Read the model definition and answer for the solid it produces. Units are mm, in the model's axes. Give positions to 0.01 mm unless a question says otherwise; leave off trailing zeros. Order: outer loops, then holes, each group sorted by start corner. A loop starts at its lowest first (then second) coordinate and runs counter-clockwise, first axis right, second up.
Item 1: A cutting plane is placed at D-D (z = 13.3). Write down the section's boundary in (x, y), plus the area to 3 significant figures.
Item 2: A cutting plane is placed at C-C (y = 2). Write down the section's boundary in (x, z), plus the area to 3 significant figures.
Item 3: The mould has two halves that part along Y. Classify faces 1 (the face through (0, -6, 10)), 2 (the face through (13.32, -9.74, 11.01)): +Y half, -Y half, draft (parallel to the pull), parting line (faces both ways), or undercut.
Item 4: A cutting plane is placed at B-B (x = -13.5). Write down the section's boundary in (y, z).
Item 5: A cutting plane is placed at A-A (x = 0). Write down the section's boundary in (y, z), plus the area to 3 significant figures.
Item 6: Find the intervals of material crossed by line 1 along Y through (x, z) = (0, 10.55); line 2 along X through (y, z) = (-7, 10.9); line 3 along X through (y, z) = (13, 11), in increasing order.
Item 7: Given pin 1 Ø2 at (y, z) = (-8.5, 11) entering from -X; pin 2 Ø2 at (y, z) = (10, 11) entering from +X; pin 3 Ø1.6 at (y, z) = (12.5, 11.5) entering from -X; pin 4 Ø1.5 at (y, z) = (21, 13) entering from +X, each flat-ended and moving along its own axis, determine where each tip first touches the part or whether it passes through.
from build123d import *

# Parameters (mm, degrees)
BOSS_EXTRUDE1_DEPTH    = 2
BOSS_EXTRUDE1_2_DEPTH  = 2
BOSS_EXTRUDE1_3_DEPTH  = 2
BOSS_EXTRUDE1_4_DEPTH  = 2
BOSS_EXTRUDE1_5_DEPTH  = 2
BOSS_EXTRUDE1_6_DEPTH  = 2
BOSS_EXTRUDE1_7_DEPTH  = 2
BOSS_EXTRUDE1_8_DEPTH  = 2
BOSS_EXTRUDE1_9_DEPTH  = 2
BOSS_EXTRUDE1_10_DEPTH = 2
SKETCH3_R              = 30
SKETCH3_R_2            = 16.5
BOSS_EXTRUDE2_DEPTH    = 2
SKETCH4_R              = 2.9
BOSS_EXTRUDE3_DEPTH    = 2
SKETCH6_R              = 5
BOSS_EXTRUDE4_DEPTH    = 1
SKETCH13_R             = 4.177329345
BOSS_EXTRUDE6_DEPTH    = 2
FILLET2_R              = 0.5
SKETCH14_R             = 3
CUT_EXTRUDE1_DEPTH     = 20


with BuildPart() as part:
    # Sketch2 → Boss-Extrude1 (new body)
    with BuildSketch(Plane.XY.offset(10)):
        with BuildLine():
            Line((8.357492916, 13.704694326), (0.999285991, 3.572733706))
            Line((0.999285991, 3.572733706), (0.999663781, 1.6824161))
            Line((0.999663781, 1.6824161), (3.379039645, 2.45604795))
            Line((3.379039645, 2.45604795), (10.446460828, 12.187608075))
            ThreePointArc((10.446460828, 12.187608075), (10.160519997, 13.990635156), (8.357492916, 13.704694326))
        make_face()
    extrude(amount=BOSS_EXTRUDE1_DEPTH)


with BuildPart() as body_2:
    # Sketch2 → Boss-Extrude1 2 (new body)
    with BuildSketch(Plane.XY.offset(10)):
        with BuildLine():
            Line((0.999285991, 3.572733706), (0.996802301, 16.000199535))
            ThreePointArc((0.996802301, 16.000199535), (-0.003397534, 16.99999966), (-1.003197659, 15.999799826))
            Line((-1.003197659, 15.999799826), (-1.000713969, 3.572333996))
            Line((-1.000713969, 3.572333996), (-0.000438912, 2.196151958))
            Line((-0.000438912, 2.196151958), (0.999285991, 3.572733706))
        make_face()
    extrude(amount=BOSS_EXTRUDE1_2_DEPTH)


with BuildPart() as body_3:
    # Sketch2 → Boss-Extrude1 3 (new body)
    with BuildSketch(Plane.XY.offset(10)):
        with BuildLine():
            Line((-1.000336179, 1.68201639), (-1.000713969, 3.572333996))
            Line((-1.000713969, 3.572333996), (-8.362970151, 13.701352658))
            ThreePointArc((-8.362970151, 13.701352658), (-10.166111381, 13.986572778), (-10.451331501, 12.183431547))
            Line((-10.451331501, 12.183431547), (-3.380021082, 2.454697118))
            Line((-3.380021082, 2.454697118), (-1.000336179, 1.68201639))
        make_face()
    extrude(amount=BOSS_EXTRUDE1_3_DEPTH)


with BuildPart() as body_4:
    # Sketch2 → Boss-Extrude1 4 (new body)
    with BuildSketch(Plane.XY.offset(10)):
        with BuildLine():
            Line((-2.088800262, 0.678230847), (-3.380021082, 2.454697118))
            Line((-3.380021082, 2.454697118), (-14.819238004, 6.168996626))
            ThreePointArc((-14.819238004, 6.168996626), (-16.445658083, 5.339884727), (-15.616546184, 3.713464648))
            Line((-15.616546184, 3.713464648), (-4.177329262, -0.00083486))
            Line((-4.177329262, -0.00083486), (-2.088800262, 0.678230847))
        make_face()
    extrude(amount=BOSS_EXTRUDE1_4_DEPTH)


with BuildPart() as body_5:
    # Sketch2 → Boss-Extrude1 5 (new body)
    with BuildSketch(Plane.XY.offset(10)):
        with BuildLine():
            Line((-2.088529, -0.679065707), (-4.177329262, -0.00083486))
            Line((-4.177329262, -0.00083486), (-15.615060628, -3.71970644))
            ThreePointArc((-15.615060628, -3.71970644), (-16.443522365, -5.346457793), (-14.816771011, -6.17491953))
            Line((-14.816771011, -6.17491953), (-3.379039645, -2.45604795))
            Line((-3.379039645, -2.45604795), (-2.088529, -0.679065707))
        make_face()
    extrude(amount=BOSS_EXTRUDE1_5_DEPTH)


with BuildPart() as body_6:
    # Sketch2 → Boss-Extrude1 6 (new body)
    with BuildSketch(Plane.XY.offset(10)):
        with BuildLine():
            Line((-1.290510646, -1.776982243), (-3.379039645, -2.45604795))
            Line((-3.379039645, -2.45604795), (-10.446460828, -12.187608075))
            ThreePointArc((-10.446460828, -12.187608075), (-10.160519997, -13.990635156), (-8.357492916, -13.704694326))
            Line((-8.357492916, -13.704694326), (-1.290071734, -3.973134201))
            Line((-1.290071734, -3.973134201), (-1.290510646, -1.776982243))
        make_face()
    extrude(amount=BOSS_EXTRUDE1_6_DEPTH)


with BuildPart() as body_7:
    # Sketch2 → Boss-Extrude1 7 (new body)
    with BuildSketch(Plane.XY.offset(10)):
        with BuildLine():
            Line((1.294063412, -15.999741695), (1.291659732, -3.972618229))
            Line((1.291659732, -3.972618229), (0.000438912, -2.196151958))
            Line((0.000438912, -2.196151958), (-1.290071734, -3.973134201))
            Line((-1.290071734, -3.973134201), (-1.287668054, -16.000257666))
            ThreePointArc((-1.287668054, -16.000257666), (0.003455665, -17.290865413), (1.294063412, -15.999741695))
        make_face()
    extrude(amount=BOSS_EXTRUDE1_7_DEPTH)


with BuildPart() as body_8:
    # Sketch2 → Boss-Extrude1 8 (new body)
    with BuildSketch(Plane.XY.offset(10)):
        with BuildLine():
            Line((10.451331501, -12.183431547), (3.380021082, -2.454697118))
            Line((3.380021082, -2.454697118), (1.29122082, -1.776466271))
            Line((1.29122082, -1.776466271), (1.291659732, -3.972618229))
            Line((1.291659732, -3.972618229), (8.362970151, -13.701352658))
            ThreePointArc((8.362970151, -13.701352658), (10.166111381, -13.986572778), (10.451331501, -12.183431547))
        make_face()
    extrude(amount=BOSS_EXTRUDE1_8_DEPTH)


with BuildPart() as body_9:
    # Sketch2 → Boss-Extrude1 9 (new body)
    with BuildSketch(Plane.XY.offset(10)):
        with BuildLine():
            Line((15.616546184, -3.713464648), (4.177329262, 0.00083486))
            Line((4.177329262, 0.00083486), (2.088800262, -0.678230847))
            Line((2.088800262, -0.678230847), (3.380021082, -2.454697118))
            Line((3.380021082, -2.454697118), (14.819238004, -6.168996626))
            ThreePointArc((14.819238004, -6.168996626), (16.445658083, -5.339884727), (15.616546184, -3.713464648))
        make_face()
    extrude(amount=BOSS_EXTRUDE1_9_DEPTH)


with BuildPart() as body_10:
    # Sketch2 → Boss-Extrude1 10 (new body)
    with BuildSketch(Plane.XY.offset(10)):
        with BuildLine():
            Line((14.816771011, 6.17491953), (3.379039645, 2.45604795))
            Line((3.379039645, 2.45604795), (2.088529, 0.679065707))
            Line((2.088529, 0.679065707), (4.177329262, 0.00083486))
            Line((4.177329262, 0.00083486), (15.615060628, 3.71970644))
            ThreePointArc((15.615060628, 3.71970644), (16.443522365, 5.346457793), (14.816771011, 6.17491953))
        make_face()
    extrude(amount=BOSS_EXTRUDE1_10_DEPTH)


with BuildPart() as body_11:
    # Sketch3 → Boss-Extrude2 (new body)
    with BuildSketch(Plane.XY.offset(12)):
        Circle(SKETCH3_R)
        Circle(SKETCH3_R_2, mode=Mode.SUBTRACT)
    extrude(amount=-BOSS_EXTRUDE2_DEPTH)

    # Sketch4 → Boss-Extrude3 (add)
    with BuildSketch(Plane.XY.offset(12)):
        with Locations((0, 25)):
            Circle(SKETCH4_R)
        with Locations((21.650635095, -12.5)):
            Circle(SKETCH4_R)
        with Locations((-21.650635095, -12.5)):
            Circle(SKETCH4_R)
    extrude(amount=BOSS_EXTRUDE3_DEPTH)

    # Sketch6 → Boss-Extrude4 (add)
    with BuildSketch(Plane(origin=(0, 0, 11), x_dir=(-1, 0, 0), z_dir=(0, 0, -1))):
        with Locations((0, 30)):
            Circle(SKETCH6_R)
        with Locations((25.980762114, -15)):
            Circle(SKETCH6_R)
        with Locations((-25.980762114, -15)):
            Circle(SKETCH6_R)
    extrude(amount=-BOSS_EXTRUDE4_DEPTH)


    add(part.part)  # Boss-Extrude6 merges part

    add(body_3.part)  # Boss-Extrude6 merges body 3

    add(body_5.part)  # Boss-Extrude6 merges body 5

    add(body_7.part)  # Boss-Extrude6 merges body 7

    add(body_9.part)  # Boss-Extrude6 merges body 9

    add(body_2.part)  # Boss-Extrude6 merges body 2

    add(body_4.part)  # Boss-Extrude6 merges body 4

    add(body_6.part)  # Boss-Extrude6 merges body 6

    add(body_8.part)  # Boss-Extrude6 merges body 8

    add(body_10.part)  # Boss-Extrude6 merges body 10
    # Sketch13 → Boss-Extrude6 (add)
    with BuildSketch(Plane(origin=(0, 0, 10), x_dir=(-1, 0, 0), z_dir=(0, 0, -1))):
        Circle(SKETCH13_R)
    extrude(amount=-BOSS_EXTRUDE6_DEPTH)

    # Fillet2
    fillet2_edges = [body_11.edges().sort_by_distance(p)[0] for p in [
        (-1.290071734, -3.973134201, 11),
        (1.291659732, -3.972618229, 11),
        (3.380021082, -2.454697118, 11),
        (4.177329262, 0.00083486, 11),
        (3.379039645, 2.45604795, 11),
        (-3.380021082, 2.454697118, 11),
        (-4.177329262, -0.00083486, 11),
        (-3.379039645, -2.45604795, 11),
    ]]
    fillet(fillet2_edges, radius=FILLET2_R)

    # Sketch14 → Cut-Extrude1 (cut)
    with BuildSketch(Plane(origin=(0, 0, 10), x_dir=(-1, 0, 0), z_dir=(0, 0, -1))):
        Circle(SKETCH14_R)
    extrude(amount=-CUT_EXTRUDE1_DEPTH, mode=Mode.SUBTRACT)


solid = body_11.part
Response values:
1. outline: circle Ø5.8 at (-21.65, -12.5); circle Ø5.8 at (0, 25); circle Ø5.8 at (21.65, -12.5)
1. area: 79.3 mm2
2. outline: (-29.93, 10) - (-16.38, 10) - (-16.38, 12) - (-29.93, 12) - close; (-10.34, 10) - (-2.24, 10) - (-2.24, 12) - (-10.34, 12) - close; (2.24, 10) - (10.33, 10) - (10.33, 12) - (2.24, 12) - close; (16.38, 10) - (29.93, 10) - (29.93, 12) - (16.38, 12) - close
2. area: 86.6 mm2
3. face 1: draft
3. face 2: undercut
4. outline: (-26.79, 10) - (-9.49, 10) - (-9.49, 12) - (-26.79, 12) - close; (-5.75, 10) - (-3.03, 10) - (-3.03, 12) - (-5.75, 12) - close; (3.03, 10) - (5.74, 10) - (5.74, 12) - (3.03, 12) - close; (9.49, 10) - (26.79, 10) - (26.79, 12) - (9.49, 12) - close
5. outline: (-30, 10) - (-3, 10) - (-3, 12) - (-30, 12) - close; (3, 10) - (30, 10) - (30, 11) - (35, 11) - (35, 12) - (27.9, 12) - (27.9, 14) - (22.1, 14) - (22.1, 12) - (3, 12) - close
5. area: 125 mm2
6. line 1: y = -30 to -3, 3 to 30
6. line 2: x = -29.17 to -14.94, -6.68 to -3.49, -1.29 to 1.29, 3.49 to 6.68, 14.94 to 29.17
6. line 3: x = -27.04 to -7.85, -1 to 1, 7.85 to 27.04
7. pin 1: stops at x = -29.05
7. pin 2: stops at x = 28.62
7. pin 3: stops at x = -27.62
7. pin 4: passes through
